Geometry: final body of the model. Coordinates: model frame, mm. Face numbers are marked on the shaded views. Coordinates: 2 decimals unless noted, no trailing zeros. Order: outer loops, then holes, each group sorted by start corner. A loop starts at its lowest first (then second) coordinate and runs counter-clockwise, first axis right, second up. Notation, with made-up numbers: M -33,84.5 L 26,84.5 A29 cw 26,116.5 Z; hole C 88.25,86.5 d6. An arc over 180 degrees is marked long. Write item = value, one per line. Start each with the question number.
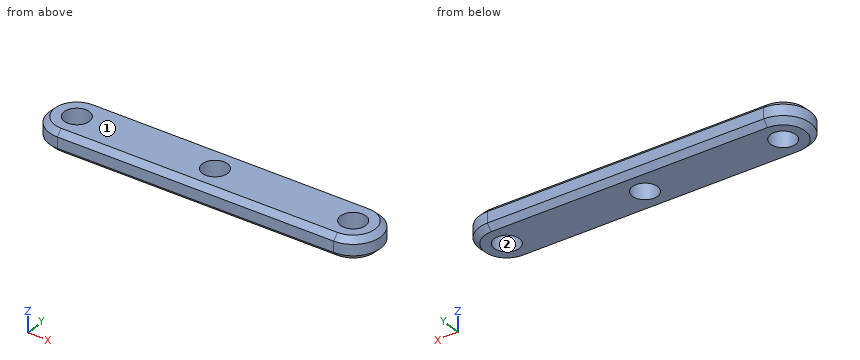
```python
from build123d import *

# Parameters (mm, degrees)
SKETCH1_R           = 2.3
BOSS_EXTRUDE1_DEPTH = 4
CHAMFER1_SIZE       = 1


with BuildPart() as part:
    # Sketch1 → Boss-Extrude1 (new body)
    with BuildSketch(Plane.XY):
        with BuildLine():
            Line((50, 5), (0, 5))
            ThreePointArc((0, 5), (-5, 0), (0, -5))
            Line((0, -5), (50, -5))
            ThreePointArc((50, -5), (55, 0), (50, 5))
        make_face()
        with Locations((25, 0)):
            Circle(SKETCH1_R, mode=Mode.SUBTRACT)
        Circle(SKETCH1_R, mode=Mode.SUBTRACT)
        with Locations((50, 0)):
            Circle(SKETCH1_R, mode=Mode.SUBTRACT)
    extrude(amount=BOSS_EXTRUDE1_DEPTH)

    # Chamfer1
    chamfer1_edges = [part.edges().sort_by_distance(p)[0] for p in [
        (-5, 0, 0),
        (25, 5, 0),
        (55, 0, 0),
        (25, -5, 0),
        (55, 0, 4),
        (25, 5, 4),
        (-5, 0, 4),
        (25, -5, 4),
    ]]
    chamfer(chamfer1_edges, length=CHAMFER1_SIZE)


solid = part.part
```
Item 1: Section query C-C on z = 0.5. Output: boundary loops of the cut face in (x, y), and give its area (3 significant figures).
Item 2: Draft query along Y for the marked faces 1 and 2. Return one class per face: pulls with the +Y half, pulls with the -Y half, needs draft (parallel to the pull), parting line crosses it, or undercut.
Item 3: Section query B-B on x = 25. Output: boundary loops of the cut face in (y, z).
Item 4: Material intervals for probe 1 along X at (y, z) = (-1, 1.9); probe 2 along Y at (x, z) = (25, 2.3); probe 3 along X at (y, z) = (1.5, 1.4), sorted ascending. Write a range as [from, to].
Item 5: Section query D-D on x = 43. Output: boundary loops of the cut face in (y, z).
Item 6: First-contact query: pin 1 (1.5 mm diameter, centred on y = 2, z = 1.5, fed in from -X); pin 2 (1 mm diameter, centred on y = 1, z = 1, fed in from -X). Flat tips, straight axial feed; report the tip coordinate or a pass-through.
Item 7: Section query A-A on y = 0. Output: boundary loops of the cut face in (x, z).
Ans:
q1.outline = M 0,-4.5 L 50,-4.5 A4.5 ccw 50,4.5 L 0,4.5 A4.5 ccw Z; hole C 0,0 d4.6; hole C 25,0 d4.6; hole C 50,0 d4.6
q1.area = 464 mm^2
q2.face_1 = needs draft
q2.face_2 = undercut
q3.outline = M -5,1 L -4,0 L -2.3,0 L -2.3,4 L -4,4 L -5,3 Z; M 2.3,0 L 4,0 L 5,1 L 5,3 L 4,4 L 2.3,4 Z
q4.probe_1 = [-4.9, -2.07], [2.07, 22.93], [27.07, 47.93], [52.07, 54.9]
q4.probe_2 = [-5, -2.3], [2.3, 5]
q4.probe_3 = [-4.77, -1.74], [1.74, 23.26], [26.74, 48.26], [51.74, 54.77]
q5.outline = M -5,1 L -4,0 L 4,0 L 5,1 L 5,3 L 4,4 L -4,4 L -5,3 Z
q6.pin_1 = -4.84
q6.pin_2 = -4.97
q7.outline = M -5,1 L -4,0 L -2.3,0 L -2.3,4 L -4,4 L -5,3 Z; M 2.3,0 L 22.7,0 L 22.7,4 L 2.3,4 Z; M 27.3,0 L 47.7,0 L 47.7,4 L 27.3,4 Z; M 52.3,0 L 54,0 L 55,1 L 55,3 L 54,4 L 52.3,4 Z
